Input: part model. Units: mm. Frame: model coordinates. Face numbers are marked on the shaded views. Coordinates: 2 decimals unless noted, no trailing zeros. Order: outer loops, then holes, each group sorted by start corner. A loop starts at its lowest first (then second) coordinate and runs counter-clockwise, first axis right, second up. Notation, with made-up numbers: (-1.5, -7) - (27.5, -7) arc R23 cw to (27.5, 18) - close; hole circle Ø8 at (42.25, -1.75). An arc over 180 degrees is marked (long way). One line per question, with ' | ' between items.
from build123d import *

# Parameters (mm, degrees)
F0_W     = 203.2
F0_H     = 203.2
F1_DEPTH = 19.05
F2_W     = 165.1
F2_H     = 165.1
F3_DEPTH = 19.051
F5_DEPTH = 19.051


with BuildPart() as f1:
    # F0 (on Top) → F1 (new body)
    with BuildSketch(Plane.XY):
        with Locations((-20.2645299196, 37.1341121554)):
            Rectangle(F0_W, F0_H)
    extrude(amount=F1_DEPTH)

    # F2 (on face) → F3 (cut, through all)
    with BuildSketch(Plane.XY.offset(19.05)):
        with Locations((-20.2645299196, 37.1341121554)):
            Rectangle(F2_W, F2_H)
    extrude(amount=-F3_DEPTH, mode=Mode.SUBTRACT)

    # F4 (on face) → F5 (cut, through all)
    with BuildSketch(Plane.XY.offset(19.05)):
        with BuildLine():
            ThreePointArc((-107.3236708058, -54.3133095216), (-111.6306122296, -51.3469424483), (-112.8665581212, -56.4284300055))
            ThreePointArc((-112.8665581212, -56.4284300055), (-109.366729382, -57.2796765948), (-107.3236708058, -54.3133095216))
        make_face()
        with BuildLine():
            ThreePointArc((73.6524293098, 128.0401629025), (73.4153509009, 129.2440074624), (72.739521137, 130.2680689969))
            ThreePointArc((72.739521137, 130.2680689969), (67.5395077186, 126.8363183426), (73.6524293098, 128.0401629025))
        make_face()
    extrude(amount=-F5_DEPTH, mode=Mode.SUBTRACT)


solid = f1.part
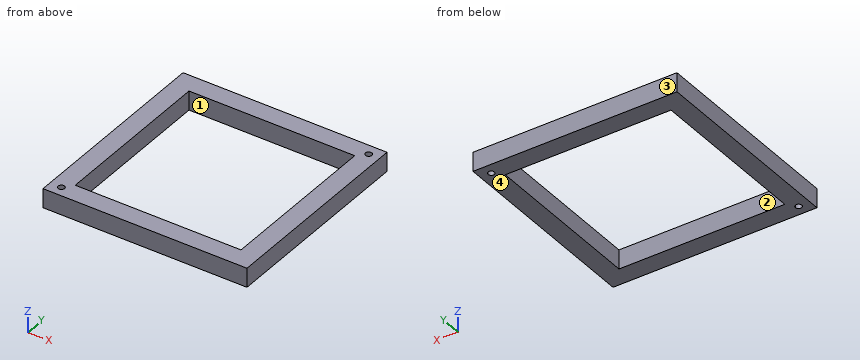
Item 1: Draft query along Y for the marked faces 1, 2, 3 and 4. Return one class per face: released by +Y, released by -Y, zero draft, split by the parting line, or undercut.
Data:
face 1: undercut | face 2: undercut | face 3: released by +Y | face 4: zero draft
Item 2: Contact query for a flat-ended pin moving along its axis: P1, Ø12, axis at x = 3.5, y = -39.5, coming from the -Z side. Output: stop coordinate, or through.
Data:
P1: z = 0
Item 3: Section A-A on y = 61. Return the cut outline in (x, z).
Data:
outline: (-121.86, 0) - (-102.81, 0) - (-102.81, 19.05) - (-121.86, 19.05) - close; (62.29, 0) - (81.34, 0) - (81.34, 19.05) - (62.29, 19.05) - close
Item 4: Ray query, line 1 (Y direction, x = 34, z = 4.25); line 2 (X direction, y = 94, z = 17); line 3 (Y direction, x = -111, z = 5). Return the intervals inside material, ascending.
Data:
line 1: -64.47 to -45.42, 119.68 to 138.73 | line 2: -121.86 to -102.81, 62.29 to 81.34 | line 3: -64.47 to -57.45, -51.18 to 138.73
Item 5: Section B-B on x = -4. Return the cut outline in (y, z).
Data:
outline: (-64.47, 0) - (-45.42, 0) - (-45.42, 19.05) - (-64.47, 19.05) - close; (119.68, 0) - (138.73, 0) - (138.73, 19.05) - (119.68, 19.05) - close
Item 6: Section C-C on z = 11. Return the cut outline in (x, y) (3 decimals), and give its area (3 significant figures).
Data:
outline: (-121.865, -64.466) - (81.335, -64.466) - (81.335, 138.734) - (-121.865, 138.734) - close; hole circle Ø6.35 at (-110.499, -54.313); hole (-102.815, -45.416) - (62.285, -45.416) - (62.285, 119.684) - (-102.815, 119.684) - close; hole circle Ø6.35 at (70.477, 128.04) | area: 14,000 mm^2
